Work out the finished part from the listing and answer in its coordinate system (mm). Face numbers are marked on the shaded views. A direction names the side the tool comes from. Round coordinates to 2 decimals unless told otherwise and drop trailing zeros. Order: outer loops, then holes, each group sorted by start corner. A loop starts at its lowest first (then second) coordinate and runs counter-clockwise, first axis right, second up. Notation, with made-up numbers: (52, 15.5) - (101, 15.5) arc R13 ccw to (101, 37.5) - close; hole circle Ø9 at (77, 84.25). An arc over 180 degrees is marked (long way). Use one line per item in the form item = value. Start each with the question number.
Q1. The part is cut by section D-D on x = -4.5. Determine the outline of the cut face in (y, z).
Q2. Find the intervals of material crossed by line 1 (Y direction, x = 22.54, z = 1.1); line 2 (Y direction, x = -22.54, z = 4); line 3 (Y direction, x = 28.5, z = 10.5), in increasing order. Write a range as [from, to].
Q3. The part is cut by section B-B on y = -1. Determine the outline of the cut face in (x, z), plus the area to 3 significant figures.
Q4. Given P1, Ø0.9, axis at x = -16.5, z = -10, coming from the -Y side; P2, Ø4.5, axis at x = -26.5, z = 6.5, coming from the -Y side; P3, Ø4.5, axis at x = 4.5, z = -10.45, coming from the -Y side, each flat-ended and moving along its own axis, determine where each tip first touches the part or whether it passes through.
Q5. The part is cut by section C-C on z = -2.45. Determine the outline of the cut face in (x, y).
Q6. Which of the six approach directions +Z, -Z, +X, -X, +Y, -Y give full straight-line access (tool end or side, diameter ignored) to the marked faces 1, 2 and 3?
Q7. For a pull along X with two mould halves and no side action, classify the marked faces 4, 5, 6 and 7 as +X half, -X half, draft (parallel to the pull), parting line (faces both ways), or undercut.
Q8. The part is cut by section A-A on z = 6.5. Determine the outline of the cut face in (x, y).
from build123d import *

# Parameters (mm, degrees)
PAD_DEPTH           = 2
PAD001_DEPTH        = 3
PAD002_DEPTH        = 3.6
PAD003_DEPTH        = 5
SKETCH004_W         = 63
SKETCH004_H         = 17.5
POCKET_DEPTH        = 11.7
PAD004_DEPTH        = 18
HOLE_D              = 3.3
HOLE_DEPTH          = 24.00858
HOLE_CSINK_D        = 6
HOLE_CSINK_ANGLE    = 90
HOLE_TIPS_R         = 1.65
SKETCH010_R         = 1.75
POCKET001_DEPTH     = 5
HOLE001_D           = 3.3
HOLE001_DEPTH       = 24.00858
HOLE001_CSINK_D     = 6
HOLE001_CSINK_ANGLE = 90
HOLE001_TIPS_R      = 1.65
SKETCH012_R         = 1.75
POCKET002_DEPTH     = 5
SKETCH013_R         = 1.75
POCKET003_DEPTH     = 35.001
POCKET004_DEPTH     = 2.5


with BuildPart() as part:
    # Sketch → Pad (new body)
    with BuildSketch(Plane.XY):
        Polygon((-31.5, 17.5), (31.5, 17.5), (31.5, -17.5), (16.5, -17.5), (16.5, -3e-05), (8.25, 14.289419), (-8.25, 14.289419), (-16.5, 0), (-16.5, -17.5), (-31.5, -17.5), align=None)
    extrude(amount=PAD_DEPTH)

    # Sketch001 (on Face12 of Pad) → Pad001 (join)
    with BuildSketch(Plane.XY.offset(2)):
        with BuildLine():
            ThreePointArc((10.25, -3e-05), (1.5e-05, 10.25), (-10.25, 0))
            Line((-16.5, 0), (-10.25, 0))
            Line((-16.5, -17.5), (-16.5, 0))
            Line((-16.5, -17.5), (-31.5, -17.5))
            Line((-31.5, -17.5), (-31.5, 17.5))
            Line((-31.5, 17.5), (31.5, 17.5))
            Line((31.5, 17.5), (31.5, -17.5))
            Line((31.5, -17.5), (16.5, -17.5))
            Line((16.5, -17.5), (16.5, -3e-05))
            Line((10.25, -3e-05), (16.5, -3e-05))
        make_face()
    extrude(amount=PAD001_DEPTH)

    # Sketch002 (on Face20 of Pad001) → Pad002 (join)
    with BuildSketch(Plane.XY.offset(5)):
        Polygon((16.5, 0), (8.25, 14.289419), (-8.25, 14.289419), (-16.5, 0), (-16.5, -17.5), (-31.5, -17.5), (-31.5, 17.5), (31.5, 17.5), (31.5, -17.5), (16.5, -17.5), align=None)
    extrude(amount=PAD002_DEPTH)

    # Sketch003 (on Face30 of Pad002) → Pad003 (join)
    with BuildSketch(Plane.XY.offset(8.6)):
        with BuildLine():
            Line((-31.5, 17.5), (31.5, 17.5))
            Line((31.5, 17.5), (31.5, -17.5))
            Line((31.5, -17.5), (16.5, -17.5))
            Line((16.5, -17.5), (16.5, 0))
            Line((16.5, 0), (13.25, 0))
            ThreePointArc((13.25, 0), (0, 13.25), (-13.25, 0))
            Line((-16.5, 0), (-13.25, 0))
            Line((-16.5, -17.5), (-16.5, 0))
            Line((-16.5, -17.5), (-31.5, -17.5))
            Line((-31.5, -17.5), (-31.5, 17.5))
        make_face()
    extrude(amount=PAD003_DEPTH)

    # Sketch004 (on Face40 of Pad003) → Pocket (cut)
    with BuildSketch(Plane.XY.offset(13.6)):
        with Locations((0, -8.75)):
            Rectangle(SKETCH004_W, SKETCH004_H)
    extrude(amount=-POCKET_DEPTH, mode=Mode.SUBTRACT)

    # Sketch008 (on Face1 of Pocket) → Pad004 (join)
    with BuildSketch(Plane(origin=(0, 0, 0), x_dir=(1, 0, 0), z_dir=(0, 0, -1))):
        Polygon((-8.25, -14.289419), (8.25, -14.289419), (14.767953, -2.99997), (17.767953, -3), (8.25, -17.5), (-8.25, -17.5), (-17.767949, -3), (-14.767949, -3), align=None)
    extrude(amount=PAD004_DEPTH)

    # Hole
    with Locations(Plane(origin=(0, 17.5, 0), x_dir=(-1, 0, 0), z_dir=(0, 1, 0))):
        with Locations((0, -2.45), (-4.5, -10.45), (4.5, -10.45)):
            CounterSinkHole(HOLE_D / 2, HOLE_CSINK_D / 2, depth=HOLE_DEPTH, counter_sink_angle=HOLE_CSINK_ANGLE)

    # Hole tips → Hole tip 1 section 0
    with BuildSketch(Plane(origin=(0, -6.50858, 0), x_dir=(-1, 0, 0), z_dir=(0, 1, 0)), mode=Mode.PRIVATE) as hole_tip_1_s0:
        with Locations((0, -2.45)):
            Circle(HOLE_TIPS_R)
    loft([hole_tip_1_s0.sketch, Vertex(0, -7.5, -2.45)], mode=Mode.SUBTRACT)

    # Hole tips → Hole tip 2 section 0
    with BuildSketch(Plane(origin=(0, -6.50858, 0), x_dir=(-1, 0, 0), z_dir=(0, 1, 0)), mode=Mode.PRIVATE) as hole_tip_2_s0:
        with Locations((-4.5, -10.45)):
            Circle(HOLE_TIPS_R)
    loft([hole_tip_2_s0.sketch, Vertex(4.5, -7.5, -10.45)], mode=Mode.SUBTRACT)

    # Hole tips → Hole tip 3 section 0
    with BuildSketch(Plane(origin=(0, -6.50858, 0), x_dir=(-1, 0, 0), z_dir=(0, 1, 0)), mode=Mode.PRIVATE) as hole_tip_3_s0:
        with Locations((4.5, -10.45)):
            Circle(HOLE_TIPS_R)
    loft([hole_tip_3_s0.sketch, Vertex(-4.5, -7.5, -10.45)], mode=Mode.SUBTRACT)

    # Sketch010 → Pocket001 (cut)
    with BuildSketch(Plane.XY.offset(1.9)):
        with Locations((-22.54, 24.3)):
            Circle(SKETCH010_R)
        with Locations((7.79, 24.3)):
            Circle(SKETCH010_R)
    extrude(amount=-POCKET001_DEPTH, mode=Mode.SUBTRACT)

    # Hole001
    with Locations(Plane.XY.offset(13.6)):
        with Locations((-22.54, 10.7), (22.54, 10.7)):
            CounterSinkHole(HOLE001_D / 2, HOLE001_CSINK_D / 2, depth=HOLE001_DEPTH, counter_sink_angle=HOLE001_CSINK_ANGLE)

    # Hole001 tips → Hole001 tip 1 section 0
    with BuildSketch(Plane.XY.offset(-10.40858), mode=Mode.PRIVATE) as hole001_tip_1_s0:
        with Locations((-22.54, 10.7)):
            Circle(HOLE001_TIPS_R)
    loft([hole001_tip_1_s0.sketch, Vertex(-22.54, 10.7, -11.4)], mode=Mode.SUBTRACT)

    # Hole001 tips → Hole001 tip 2 section 0
    with BuildSketch(Plane.XY.offset(-10.40858), mode=Mode.PRIVATE) as hole001_tip_2_s0:
        with Locations((22.54, 10.7)):
            Circle(HOLE001_TIPS_R)
    loft([hole001_tip_2_s0.sketch, Vertex(22.54, 10.7, -11.4)], mode=Mode.SUBTRACT)

    # Sketch012 (on Face6 of Hole001) → Pocket002 (cut)
    with BuildSketch(Plane.XY.offset(1.9)):
        with Locations((-22.54, -10.7)):
            Circle(SKETCH012_R)
        with Locations((22.54, -10.7)):
            Circle(SKETCH012_R)
    extrude(amount=-POCKET002_DEPTH, mode=Mode.SUBTRACT)

    # Sketch013 (on Face43 of Pocket002) → Pocket003 (cut, through all)
    with BuildSketch(Plane(origin=(0, 17.5, 0), x_dir=(-1, 0, 0), z_dir=(0, 1, 0))):
        with Locations((-26.5, 6.5)):
            Circle(SKETCH013_R)
        with Locations((26.5, 6.5)):
            Circle(SKETCH013_R)
    extrude(amount=-POCKET003_DEPTH, mode=Mode.SUBTRACT)

    # Sketch014 (on Face44 of Pocket003) → Pocket004 (cut)
    with BuildSketch(Plane(origin=(0, 17.5, 0), x_dir=(-1, 0, 0), z_dir=(0, 1, 0))):
        Polygon((-26.5, 3.3), (-23.728719, 4.9), (-23.728719, 8.1), (-26.5, 9.7), (-29.271281, 8.1), (-29.271281, 4.9), align=None)
        Polygon((29.271281, 4.9), (29.271281, 8.1), (26.5, 9.7), (23.728719, 8.1), (23.728719, 4.9), (26.5, 3.3), align=None)
    extrude(amount=-POCKET004_DEPTH, mode=Mode.SUBTRACT)


solid = part.part
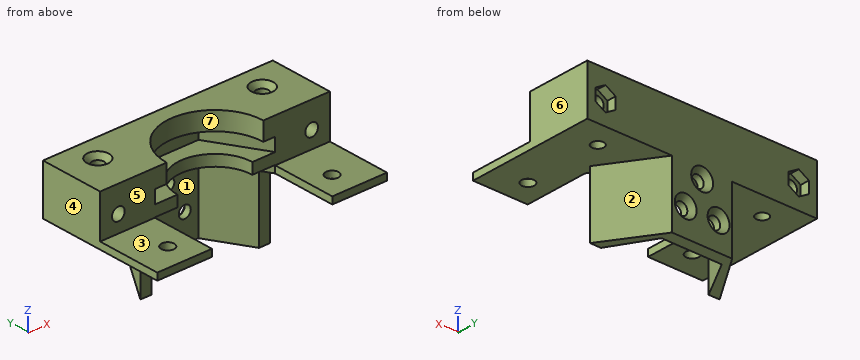
Found:
q1.outline = (9.21, 2) - (14.29, 2) - (14.29, -8.8) - (16.15, -8.8) - (17.5, -7.45) - (17.5, 13.6) - (12.46, 13.6) - (12.46, 8.6) - (14.29, 8.6) - (14.29, 5) - (9.21, 5) - close; (14.29, -18) - (17.5, -18) - (17.5, -13.45) - (16.15, -12.1) - (14.29, -12.1) - close
q2.line_1 = [-17.5, -12.45], [-8.95, 9.05], [12.35, 17.5]
q2.line_2 = [0, 9.05], [12.35, 17.5]
q2.line_3 = [0, 17.5]
q3.outline = (-31.5, 0) - (-16.5, 0) - (-16.5, 1.9) - (-31.5, 1.9) - close; (16.5, 0) - (31.5, 0) - (31.5, 1.9) - (16.5, 1.9) - close
q3.area = 57.0 mm²
q4.P1 = 3
q4.P2 = 0
q4.P3 = 14.29
q5.outline = (-17.77, 3) - (-14.77, 3) - (-8.25, 14.29) - (-1.65, 14.29) - (-1.65, 16.15) - (-3, 17.5) - (-8.25, 17.5) - close; (1.65, 14.29) - (8.25, 14.29) - (14.77, 3) - (17.77, 3) - (8.25, 17.5) - (3, 17.5) - (1.65, 16.15) - close
q6.face_1 = -Z, -Y
q6.face_2 = -Z, +X, +Y
q6.face_3 = +Z, +X, -X, -Y
q7.face_4 = -X half
q7.face_5 = draft
q7.face_6 = +X half
q7.face_7 = undercut
q8.outline = (-31.5, 0) - (-28.25, 0) - (-28.25, 15) - (-29.27, 15) - (-29.27, 17.5) - (-31.5, 17.5) - close; (-24.75, 0) - (-16.5, 0) - (-8.25, 14.29) - (8.25, 14.29) - (16.5, 0) - (24.75, 0) - (24.75, 15) - (23.73, 15) - (23.73, 17.5) - (-23.73, 17.5) - (-23.73, 15) - (-24.75, 15) - close; (28.25, 0) - (31.5, 0) - (31.5, 17.5) - (29.27, 17.5) - (29.27, 15) - (28.25, 15) - close; hole circle Ø3.3 at (-22.54, 10.7); hole circle Ø3.3 at (22.54, 10.7)
